Source: CAD feature listing. Evaluate the final solid. Frame: model axes, mm. Face numbers are marked on the shaded views. A direction names the side the tool comes from. Give positions to 0.01 mm unless a question says otherwise; leave off trailing zeros. Order: outer loops, then holes, each group sorted by start corner. A loop starts at its lowest first (then second) coordinate and runs counter-clockwise, first axis right, second up.
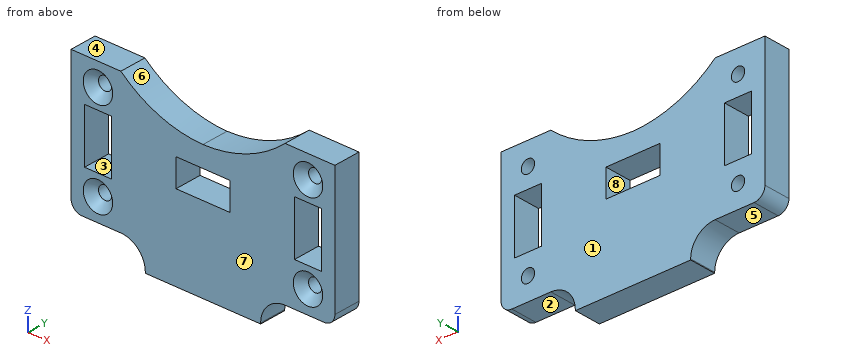
```python
from build123d import *

# Parameters (mm, degrees)
SKETCH1_R           = 1.5621
SKETCH1_W           = 6.35
SKETCH1_H           = 12.7
SKETCH1_W_2         = 12.7
SKETCH1_H_2         = 6.477
BOSS_EXTRUDE1_DEPTH = 6.35
FILLET1_R           = 2.54
CHAMFER1_SIZE       = 1.905


with BuildPart() as part:
    # Sketch1 → Boss-Extrude1 (new body)
    with BuildSketch(Plane(origin=(0, 0, 0), x_dir=(1, 0, 0), z_dir=(0, 1, 0))):
        with BuildLine():
            Line((13.568067648, 22.312647987), (-13.568067648, 22.312647987))
            Line((-13.568067648, 22.312647987), (-13.568067648, 22.095526842))
            ThreePointArc((-13.568067648, 22.095526842), (-15.25275396, 18.028334299), (-19.319946504, 16.343647987))
            Line((-19.319946504, 16.343647987), (-31.0388, 16.343647987))
            Line((-31.0388, 16.343647987), (-31.0388, -16.343647987))
            Line((-31.0388, -16.343647987), (-29.684698321, -16.343647987))
            Line((-29.684698321, -16.343647987), (-19.319946504, -16.343647987))
            ThreePointArc((-19.319946504, -16.343647987), (-10.344922534, -10.823696712), (0, -8.822823132))
            ThreePointArc((0, -8.822823132), (10.344922534, -10.823696712), (19.319946504, -16.343647987))
            Line((19.319946504, -16.343647987), (29.684698321, -16.343647987))
            Line((29.684698321, -16.343647987), (31.0388, -16.343647987))
            Line((31.0388, -16.343647987), (31.0388, 16.343647987))
            Line((31.0388, 16.343647987), (19.319946504, 16.343647987))
            ThreePointArc((19.319946504, 16.343647987), (15.25275396, 18.028334299), (13.568067648, 22.095526842))
            Line((13.568067648, 22.095526842), (13.568067648, 22.312647987))
        make_face()
        with Locations((-24.709647151, 11.044056729)):
            Circle(SKETCH1_R, mode=Mode.SUBTRACT)
        with Locations((-24.709647151, -11.044056729)):
            Circle(SKETCH1_R, mode=Mode.SUBTRACT)
        with Locations((24.709647151, 11.044056729)):
            Circle(SKETCH1_R, mode=Mode.SUBTRACT)
        with Locations((24.709647151, -11.044056729)):
            Circle(SKETCH1_R, mode=Mode.SUBTRACT)
        with Locations((24.6888, -0.068443271)):
            Rectangle(SKETCH1_W, SKETCH1_H, mode=Mode.SUBTRACT)
        with Locations((-24.6888, -0.068443271)):
            Rectangle(SKETCH1_W, SKETCH1_H, mode=Mode.SUBTRACT)
        with Locations((0, -0.737852013)):
            Rectangle(SKETCH1_W_2, SKETCH1_H_2, mode=Mode.SUBTRACT)
    extrude(amount=BOSS_EXTRUDE1_DEPTH)

    # Fillet1
    fillet1_edges = [part.edges().sort_by_distance(p)[0] for p in [
        (-31.0388, 3.175, -16.343647987),
        (31.0388, 3.175, -16.343647987),
    ]]
    fillet(fillet1_edges, radius=FILLET1_R)

    # Chamfer1
    chamfer1_edges = [part.edges().sort_by_distance(p)[0] for p in [
        (-26.271747151, 0, -11.044056729),
        (-26.271747151, 0, 11.044056729),
        (23.147547151, 0, -11.044056729),
        (23.147547151, 0, 11.044056729),
    ]]
    chamfer(chamfer1_edges, length=CHAMFER1_SIZE)


solid = part.part
```
1) Material intervals for L1, parallel to X at y = 2.5, z = 2; L2, parallel to X at y = 1, z = -3; L3, parallel to X at y = 5.5, z = 14, sorted ascending.
Report:
L1: x = -31.04 to -27.86, -21.51 to -6.35, 6.35 to 21.51, 27.86 to 31.04
L2: x = -31.04 to -27.86, -21.51 to 21.51, 27.86 to 31.04
L3: x = -31.04 to -16.34, 16.34 to 31.04
2) Section query C-C, the plane y = 0.75. Count the separate pieces of the cut face and the enclosed holes in it, and give its area (3 significant figures).
Report:
separate pieces: 1
enclosed holes: 7
area: 1,670 mm2
3) Section query B-B, the plane x = 1.5. Return the cut outline in (y, z).
Report:
outline: (0, -22.31) - (6.35, -22.31) - (6.35, -2.5) - (0, -2.5) - close; (0, 3.98) - (6.35, 3.98) - (6.35, 8.88) - (0, 8.88) - close
4) Pin query (flat end, axial travel): pin 1 (1 mm diameter, centred on y = 1, z = -18.5, fed in from +X); pin 2 (1.9 mm diameter, centred on x = -2, y = 2.5, fed in from +Z); pin 3 (3 mm diameter, centred on x = -24, y = 4.5, fed in from -Z). Return the tip coordinate at first contact, or that it passes through.
Report:
pin 1: stops at x = 15.28
pin 2: stops at z = 9
pin 3: stops at z = -16.34
5) Reachability of the marked faces 4, 5, 6, 7 and 8 from +Z, -Z, +X, -X, +Y, -Y: full face, straight path, thin tool, end or side. Return the list, or none.
Report:
face 4: +Z, +X, -X, +Y, -Y
face 5: -Z, -X, +Y, -Y
face 6: +Z, +Y, -Y
face 7: +Z, -Z, +X, -X, -Y
face 8: +Y, -Y
6) Section query A-A, the plane z = 0. Return the cut outline in (x, y).
Report:
outline: (-31.04, 0) - (-27.86, 0) - (-27.86, 6.35) - (-31.04, 6.35) - close; (-21.51, 0) - (-6.35, 0) - (-6.35, 6.35) - (-21.51, 6.35) - close; (6.35, 0) - (21.51, 0) - (21.51, 6.35) - (6.35, 6.35) - close; (27.86, 0) - (31.04, 0) - (31.04, 6.35) - (27.86, 6.35) - close
7) Draft query along Z for the marked faces 1, 2 and 3. Return one class per face: +Z half, -Z half, draft (parallel to the pull), parting line (faces both ways), or undercut.
Report:
face 1: draft
face 2: -Z half
face 3: undercut
